```python
from build123d import *

# Parameters (mm, degrees)
SKETCH1_R           = 4.1
BOSS_EXTRUDE1_DEPTH = 19
SKETCH2_W           = 10
SKETCH2_H           = 10
BOSS_EXTRUDE2_DEPTH = 5
FILLET1_R           = 2.5
CHAMFER1_SIZE       = 1


with BuildPart() as part:
    # Sketch1 → Boss-Extrude1 (new body)
    with BuildSketch(Plane(origin=(0, 0, 0), x_dir=(1, 0, 0), z_dir=(0, 1, 0))):
        with Locations(Location((0, 0, 0), (0, 0, 270))):
            Circle(SKETCH1_R)
    extrude(amount=BOSS_EXTRUDE1_DEPTH)

    # Sketch2 → Boss-Extrude2 (add)
    with BuildSketch(Plane(origin=(0, 19, 0), x_dir=(1, 0, 0), z_dir=(0, 1, 0))):
        Rectangle(SKETCH2_W, SKETCH2_H)
    extrude(amount=BOSS_EXTRUDE2_DEPTH)

    # Fillet1
    fillet1_edges = [part.edges().sort_by_distance(p)[0] for p in [
        (5, 21.5, 5),
        (5, 21.5, -5),
        (-5, 21.5, -5),
        (-5, 21.5, 5),
    ]]
    fillet(fillet1_edges, radius=FILLET1_R)

    # Chamfer1
    chamfer1_edges = [part.edges().sort_by_distance(p)[0] for p in [
        (0, 0, -4.1),
    ]]
    chamfer(chamfer1_edges, length=CHAMFER1_SIZE)


solid = part.part
```
The listing builds one solid part. Answer for the finished solid, in the listing's coordinates (mm). A direction names the side the tool comes from. Round coordinates to 2 decimals unless told otherwise and drop trailing zeros. Loops run counter-clockwise (first coordinate to the right, second up) from the corner with the lowest first, then second, coordinate; pieces in that order, holes last.
1) Given P1, Ø1.5, axis at y = 10, z = -3.5, coming from the -X side, flat-ended and moving along its own axis, determine where the tip first touches the part or whether it passes through.
Outcome:
P1: stops at x = -3.04
2) A cutting plane is placed at A-A on z = 0. Determine the outline of the cut face in (x, y), plus the area to 3 significant figures.
Outcome:
outline: (-5, 19) - (-4.1, 19) - (-4.1, 1) - (-3.1, 0) - (3.1, 0) - (4.1, 1) - (4.1, 19) - (5, 19) - (5, 24) - (-5, 24) - close
area: 205 mm2
3) For faces 4 (the face through (4.065, 9.874, -0.534)), 5 (the face through (5, 21, 0)), determine the directions among +Z, -Z, +X, -X, +Y, -Y from which every point of the face is accessible in a straight line to the end or side of a thin tool.
Outcome:
face 4: -Y
face 5: +Z, -Z, +X, +Y, -Y
4) Consider line 1 (Y direction, x = 3.75, z = -3.75); line 2 (Z direction, x = -3.25, y = 17); line 3 (Z direction, x = -2.5, y = 7.5). Determine where each line is inside the solid, lowest interval first.
Outcome:
line 1: y = 19 to 24
line 2: z = -2.5 to 2.5
line 3: z = -3.25 to 3.25
5) A cutting plane is placed at D-D on y = 15.25. Determine the outline of the cut face in (x, z), plus the area to 3 significant figures.
Outcome:
outline: circle Ø8.2 at (0, 0)
area: 52.8 mm2
6) A cutting plane is placed at B-B on x = 0. Determine the outline of the cut face in (y, z), plus the area to 3 significant figures.
Outcome:
outline: (0, -3.1) - (1, -4.1) - (19, -4.1) - (19, -5) - (24, -5) - (24, 5) - (19, 5) - (19, 4.1) - (1, 4.1) - (0, 3.1) - close
area: 205 mm2
7) For a pull along Y with two mould halves and no side action, classify faces 1 (the face through (-4.287, 21.535, -4.248)), 2 (the face through (0, 24, 0)), 3 (the face through (0, 0, 0)) as released by +Y, released by -Y, zero draft, split by the parting line, or undercut.
Outcome:
face 1: zero draft
face 2: released by +Y
face 3: released by -Y
8) A cutting plane is placed at C-C on y = 21. Determine the outline of the cut face in (x, z).
Outcome:
outline: (-5, -2.5) arc R2.5 ccw to (-2.5, -5) - (2.5, -5) arc R2.5 ccw to (5, -2.5) - (5, 2.5) arc R2.5 ccw to (2.5, 5) - (-2.5, 5) arc R2.5 ccw to (-5, 2.5) - close
